Geometry check sheet. Reference: drawing and pictorial views, mm from the part's lowest x, y, z. Coordinates: 2 decimals unless noted, no trailing zeros. Loops run counter-clockwise (first coordinate to the right, second up) from the corner with the lowest first, then second, coordinate; pieces in that order, holes last. Notation, with made-up numbers: (82.25, 54) -> (94.25, 54) arc R18 cw to (94.25, 65) -> close; hole circle Ø8 at (-31, 80). An arc over 180 degrees is marked (long way). Use CSV: the item, a comma, the result in double quotes.
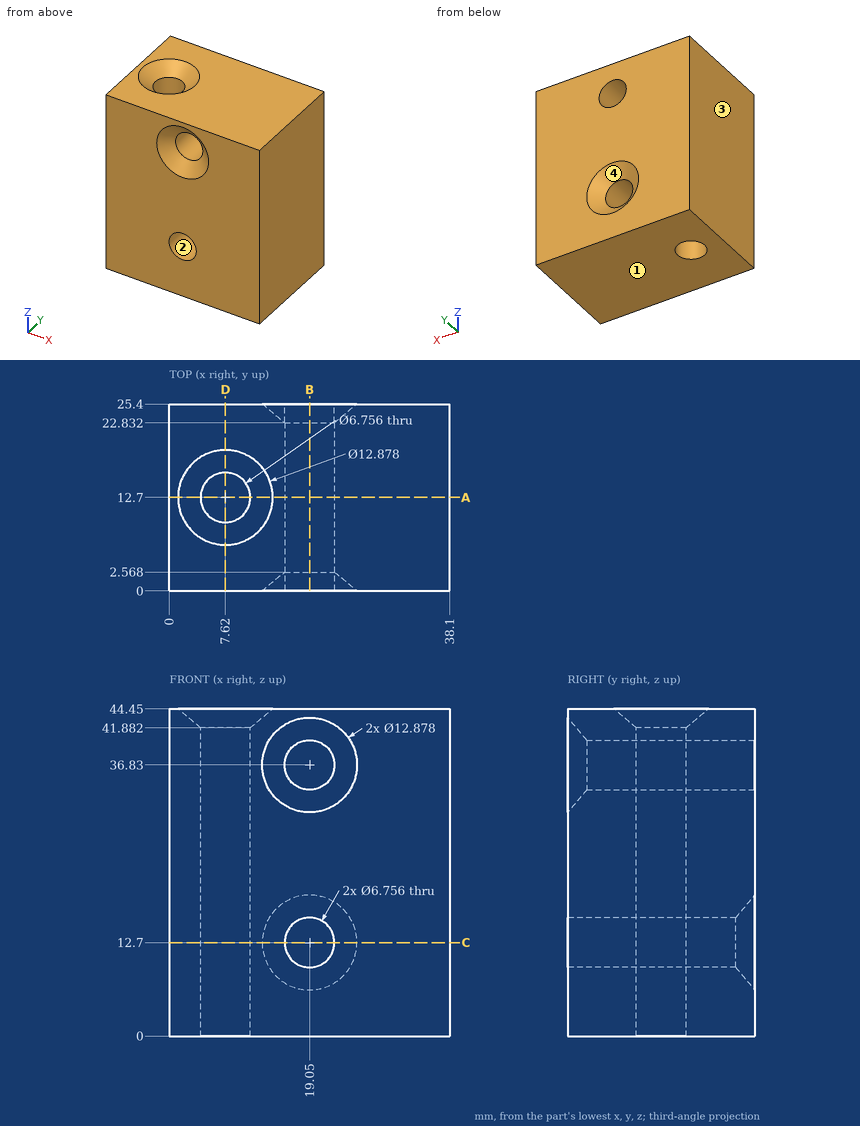
1) Thickness scan on line 1 along Z through (x, y) = (19, 21.75); line 2 along Y through (x, z) = (7.62, 18.5); line 3 along X through (y, z) = (12, 35) (1 decimal). Record the ranges inside material, lowest first. Write a range as from..to.
Answer below:
line 1,"z = 0..9.32, 16.08..33.45, 40.21..44.45"
line 2,"y = 0..9.32, 16.08..25.4"
line 3,"x = 0..4.3, 10.9..16.2, 21.9..38.1"
2) Cross-section at A-A on y = 12.7. Record the boundary of the cut face in (x, z).
Answer below:
outline,"(0, 0) -> (4.24, 0) -> (4.24, 41.88) -> (1.18, 44.45) -> (0, 44.45) -> close; (11, 0) -> (38.1, 0) -> (38.1, 44.45) -> (14.06, 44.45) -> (11, 41.88) -> close; hole circle Ø6.76 at (19.05, 12.7); hole circle Ø6.76 at (19.05, 36.83)"
3) Cross-section at B-B on x = 19.05. Record the boundary of the cut face in (y, z).
Answer below:
outline,"(0, 0) -> (25.4, 0) -> (25.4, 6.26) -> (22.83, 9.32) -> (0, 9.32) -> close; (0, 16.08) -> (22.83, 16.08) -> (25.4, 19.14) -> (25.4, 33.45) -> (2.57, 33.45) -> (0, 30.39) -> close; (0, 43.27) -> (2.57, 40.21) -> (25.4, 40.21) -> (25.4, 44.45) -> (0, 44.45) -> close"
4) Go/stop test with flat-tipped pins: pin 1 Ø1 at (x, z) = (15.5, 32.5) entering from -Y (1 decimal); pin 2 Ø9 at (x, y) = (7.62, 12.7) entering from +Z. Record where each tip stops, or that it passes through.
Answer below:
pin 1,"stops at y = 0.3"
pin 2,"stops at z = 42.82"
5) Cross-section at C-C on z = 12.7. Record the boundary of the cut face in (x, y).
Answer below:
outline,"(0, 0) -> (15.67, 0) -> (15.67, 22.83) -> (12.61, 25.4) -> (0, 25.4) -> close; (22.43, 0) -> (38.1, 0) -> (38.1, 25.4) -> (25.49, 25.4) -> (22.43, 22.83) -> close; hole circle Ø6.76 at (7.62, 12.7)"
6) Cross-section at D-D on x = 7.62. Record the boundary of the cut face in (y, z).
Answer below:
outline,"(0, 0) -> (9.32, 0) -> (9.32, 41.88) -> (6.26, 44.45) -> (0, 44.45) -> close; (16.08, 0) -> (25.4, 0) -> (25.4, 44.45) -> (19.14, 44.45) -> (16.08, 41.88) -> close"
7) Draft check along Z on the marked faces 1, 2, 3 and 4. Enter one of: released by +Z, released by -Z, zero draft, split by the parting line, or undercut.
Answer below:
face 1,"released by -Z"
face 2,"undercut"
face 3,"zero draft"
face 4,"undercut"
